```python
from build123d import *

# Parameters (mm, degrees)
BOSS_EXTRUDE1_DEPTH = 1
BOSS_EXTRUDE2_DEPTH = 0.5


with BuildPart() as part:
    # Sketch1 → Boss-Extrude1 (new body)
    with BuildSketch(Plane(origin=(0, 0, 0), x_dir=(1, 0, 0), z_dir=(0, 1, 0))):
        Polygon((5.877852523, -8.090169944), (9.510565163, 3.090169944), (0, 10), (-9.510565163, 3.090169944), (-5.877852523, -8.090169944), align=None)
        Polygon((-5.316743775, -7.690169944), (5.316743775, -7.690169944), (0, -3.9), align=None, mode=Mode.SUBTRACT)
        Polygon((5.622138751, -7.582748818), (2.153438567, -0.699694605), (9.005433722, 2.829962413), align=None, mode=Mode.SUBTRACT)
        Polygon((8.830044516, 3.090169944), (2.153438567, 3.090169944), (0.199189097, 9.360853459), align=None, mode=Mode.SUBTRACT)
        Polygon((-0.199189097, 9.360853459), (-2.153438567, 3.090169944), (-8.830044516, 3.090169944), align=None, mode=Mode.SUBTRACT)
        Polygon((-9.005433722, 2.829962413), (-2.153438567, -0.699694605), (-5.622138751, -7.582748818), align=None, mode=Mode.SUBTRACT)
    extrude(amount=BOSS_EXTRUDE1_DEPTH)

    # Sketch1_2 → Boss-Extrude2 (add)
    with BuildSketch(Plane(origin=(0, 0, 0), x_dir=(1, 0, 0), z_dir=(0, 1, 0))):
        Polygon((5.622138751, -7.582748818), (2.153438567, -0.699694605), (9.005433722, 2.829962413), align=None)
        Polygon((8.830044516, 3.090169944), (2.153438567, 3.090169944), (0.199189097, 9.360853459), align=None)
        Polygon((-0.199189097, 9.360853459), (-2.153438567, 3.090169944), (-8.830044516, 3.090169944), align=None)
        Polygon((-9.005433722, 2.829962413), (-2.153438567, -0.699694605), (-5.622138751, -7.582748818), align=None)
        Polygon((0, -3.9), (5.316743775, -7.690169944), (-5.316743775, -7.690169944), align=None)
    extrude(amount=BOSS_EXTRUDE2_DEPTH)


solid = part.part
```
Read the model definition and answer for the solid it produces. Units are mm, in the model's axes. A direction names the side the tool comes from. Give positions to 0.01 mm unless a question says otherwise; leave off trailing zeros. Order: outer loops, then holes, each group sorted by start corner. A loop starts at its lowest first (then second) coordinate and runs counter-clockwise, first axis right, second up. Notation, with made-up numbers: (23, -23.75) -> (76, -23.75) arc R12 cw to (76, -15.75) -> close; hole circle Ø9 at (23, 77.25). An arc over 180 degrees is marked (long way). One line per item, written item: value. Start each with the question number.
(1) Straight lines are drawn through the part: L1, parallel to X at y = 0.9, z = -5.5; L2, parallel to X at y = 0.55, z = 0.5; L3, parallel to Z at x = 4, y = 0.75. For each, find the intervals that lie inside material, in ascending order.
(2) The part is cut by section C-C (y = 0.25). Determine the outline of the cut face in (x, z), and give its area (3 significant figures).
(3) The part is cut by section A-A (x = -7.25). Determine the outline of the cut face in (y, z), and give its area (3 significant figures).
(4) For a pull along Z with two mould halves and no side action, classify faces 1 (the flat face through (-2.62, 0.75, 5.77)), 2 (the flat face through (0, 0, 1)), 3 (the flat face through (4.82, 0.49, -6.5)) as released by +Z, released by -Z, zero draft, split by the parting line, or undercut.
(5) The part is cut by section D-D (x = -2.5). Determine the outline of the cut face in (y, z), and give its area (3 significant figures).
(6) The part is cut by section B-B (z = 2). Determine the outline of the cut face in (x, y).
(7) A tool of negligible diameter and unlimited length cuts with its end or side. For faces 4 (the flat face through (4, 0.5, -5)), 5 (the flat face through (7.67, 0.49, 2.58)), from which of +Z, -Z, +X, -X, +Y, -Y can it reach the whole face along a straight path? Write none if from no direction.
Taken from the geometry:
1. L1: -6.19 to -5.51, -1.4 to 1.4, 5.51 to 6.19
1. L2: -8.34 to -7.92, -2.54 to 2.54, 7.92 to 8.34
1. L3: -7.09 to -6.6, -3.09 to -0.25, 4.36 to 6.75, 7.69 to 8.09
2. outline: (-9.51, -3.09) -> (0, -10) -> (9.51, -3.09) -> (5.88, 8.09) -> (-5.88, 8.09) -> close
2. area: 238 mm^2
3. outline: (0, -4.73) -> (1, -4.73) -> (1, -4.24) -> (0.5, -4.24) -> (0.5, -3.09) -> (1, -3.09) -> (1, -1.93) -> (0.5, -1.93) -> (0.5, 2.57) -> (1, 2.57) -> (1, 3.87) -> (0, 3.87) -> close
3. area: 5.78 mm^2
4. face 1: undercut
4. face 2: zero draft
4. face 3: released by -Z
5. outline: (0, -8.18) -> (1, -8.18) -> (1, -7.69) -> (0.5, -7.69) -> (0.5, -3.09) -> (1, -3.09) -> (1, 0.52) -> (0.5, 0.52) -> (0.5, 1.39) -> (1, 1.39) -> (1, 5.68) -> (0.5, 5.68) -> (0.5, 7.69) -> (1, 7.69) -> (1, 8.09) -> (0, 8.09) -> close
5. area: 12.5 mm^2
6. outline: (-7.86, 0) -> (7.86, 0) -> (7.86, 1) -> (7.44, 1) -> (7.44, 0.5) -> (2.81, 0.5) -> (2.81, 1) -> (-2.81, 1) -> (-2.81, 0.5) -> (-7.44, 0.5) -> (-7.44, 1) -> (-7.86, 1) -> close
7. face 4: +Y
7. face 5: +Z, +X, +Y, -Y
